Read the model definition and answer for the solid it produces. Units are mm, in the model's axes. Coordinates: 2 decimals unless noted, no trailing zeros. Write each loop counter-clockwise with the first axis right and the second up, starting at its lowest first coordinate (ties: lowest second). Pieces come first, ordered by that corner, then holes. Notation, with made-up numbers: (39.5, 46.25) -> (61.5, 46.25) arc R7 cw to (61.5, 56.25) -> close; hole circle Ø5 at (-31, 7.25). An arc over 180 degrees is marked (long way). One line per item, written item: value. Start each with the question number.
1. Find section B-B, the plane z = 10.16. Write down the section's boundary in (x, y).
2. Find section D-D, the plane y = -17.75. Write down the section's boundary in (x, z).
3. Find section A-A, the plane y = -13. Write down the section's boundary in (x, z), and give its area (3 significant figures).
4. Consider line 1 along Z through (x, y) = (-17.78, -13.25); line 2 along X through (y, z) = (-27.25, 13.5); line 3 along Z through (x, y) = (-16, -14). Determine where each line is inside the solid, lowest interval first.
5. For a pull along Y with two mould halves and no side action, classify faces 1 (the cylindrical face through (17.97, -14.15, 0.36)), 2 (the flat face through (-1, -30, 0)), 3 (the flat face through (-1, 0, 0)), 4 (the flat face through (-1, -15, 25.4)) as pulls with the +Y half, pulls with the -Y half, needs draft (parallel to the pull), parting line crosses it, or undercut.
6. Find section C-C, the plane x = -17.78. Write down the section's boundary in (y, z).
```python
from build123d import *

# Parameters (mm, degrees)
F0_W     = 76.2
F0_H     = 50.8
F0_R     = 6.35
F1_DEPTH = 30
F2_R     = 3
F3_DEPTH = 50.801
F4_R     = 3


with BuildPart() as f1:
    # F0 (on Front) → F1 (new body)
    with BuildSketch(Plane.XZ):
        Rectangle(F0_W, F0_H)
        with Locations((-17.78, 10.16)):
            Circle(F0_R, mode=Mode.SUBTRACT)
    extrude(amount=F1_DEPTH)

    # F2 (on face) → F3 (cut, through all)
    with BuildSketch(Plane.XY.offset(25.4)):
        with Locations((15.198684, -13)):
            Circle(F2_R)
    extrude(amount=-F3_DEPTH, mode=Mode.SUBTRACT)

    # F4
    f4_edges = [f1.edges().sort_by_distance(p)[0] for p in [
        (38.1, -15, -25.4),
    ]]
    fillet(f4_edges, radius=F4_R)


solid = f1.part
```
Answer block:
1. outline: (-38.1, -30) -> (-24.13, -30) -> (-24.13, 0) -> (-38.1, 0) -> close; (-11.43, -30) -> (38.1, -30) -> (38.1, 0) -> (-11.43, 0) -> close; hole circle Ø6 at (15.2, -13)
2. outline: (-38.1, -25.4) -> (35.1, -25.4) arc R3 ccw to (38.1, -22.4) -> (38.1, 25.4) -> (-38.1, 25.4) -> close; hole circle Ø12.7 at (-17.78, 10.16)
3. outline: (-38.1, -25.4) -> (12.2, -25.4) -> (12.2, 25.4) -> (-38.1, 25.4) -> close; (18.2, -25.4) -> (35.1, -25.4) arc R3 ccw to (38.1, -22.4) -> (38.1, 25.4) -> (18.2, 25.4) -> close; hole circle Ø12.7 at (-17.78, 10.16)
3. area: 3,440 mm2
4. line 1: z = -25.4 to 3.81, 16.51 to 25.4
4. line 2: x = -38.1 to -23.18, -12.38 to 38.1
4. line 3: z = -25.4 to 4.06, 16.26 to 25.4
5. face 1: undercut
5. face 2: pulls with the -Y half
5. face 3: pulls with the +Y half
5. face 4: needs draft
6. outline: (-30, -25.4) -> (0, -25.4) -> (0, 3.81) -> (-30, 3.81) -> close; (-30, 16.51) -> (0, 16.51) -> (0, 25.4) -> (-30, 25.4) -> close
